The model under review builds one solid part; all positions refer to its coordinate system, in mm. A direction names the side the tool comes from. Round coordinates to 2 decimals unless told otherwise and drop trailing zeros. Write each loop counter-clockwise with the first axis right and the second up, starting at its lowest first coordinate (ties: lowest second). Pieces come first, ordered by that corner, then holes. Notation, with made-up numbers: (-5.75, 68.25) - (48.25, 68.25) arc R11 cw to (48.25, 84.25) - close; hole circle Ø2 at (14.5, -17.5). An arc over 180 degrees is marked (long way). One line per question, with ' | ' between items. Start each with the question number.
```python
from build123d import *

# Parameters (mm, degrees)
F0_R = 31.75
F2_R = 42.4803799305
F4_T = -7.62
F5_R = 5.08
F6_R = 5.08
F7_R = 5.08


with BuildPart() as f3:
    # F0 (on Top) → F3 section 0
    with BuildSketch(Plane.XY):
        Circle(F0_R)
    # F2 (on offset) → F3 section 1
    with BuildSketch(Plane.XY.offset(152.4)):
        Circle(F2_R)
    loft()

    # F4
    f4_openings = [f3.faces().sort_by_distance(p)[0] for p in [
        (0, 0, 152.4),
    ]]
    offset(amount=F4_T, openings=f4_openings, kind=Kind.INTERSECTION)

    # F5
    f5_edges = [f3.edges().sort_by_distance(p)[0] for p in [
        (-42.48038, 0, 152.4),
    ]]
    fillet(f5_edges, radius=F5_R)

    # F6
    f6_edges = [f3.edges().sort_by_distance(p)[0] for p in [
        (-31.75, 0, 0),
    ]]
    fillet(f6_edges, radius=F6_R)

    # F7
    f7_edges = [f3.edges().sort_by_distance(p)[0] for p in [
        (-24.647654, 0, 7.62),
    ]]
    fillet(f7_edges, radius=F7_R)


solid = f3.part
```
1. The part is to be moulded in two halves that separate along X. For faces 1 (the face through (-8.056, -36.277, 76.839)), 2 (the face through (28.6, 9, 83.4)), 3 (the face through (0, 0, 0)), say which applies: pulls with the +X half, pulls with the -X half, needs draft (parallel to the pull), parting line crosses it, or undercut.
2. Clearance check with flat-ended pins moving along their axes: P1, Ø10, axis at y = -18.5, z = 58.5, coming from the +X side; P2, Ø5, axis at y = -17, z = 111.5, coming from the -X side; P3, Ø6, axis at y = -27.5, z = 93, coming from the -X side. State where each tip first meets the part, or that it passes through.
3. Wall thickness on line 1 along Z through (x, y) = (-17, 4); line 2 along X through (y, z) = (4, 78); line 3 along Y through (x, z) = (19.5, 15.5): over which ranges is each line inside the solid? List them lowest first. Write a range as [from, to].
4. Add section A-A, the plane x = 0. Write out the cut boundary in (y, z).
5. Add section B-B, the plane z = 61.5. Write out the cut boundary in (x, y).
6. Add section C-C, the plane z = 41.5. Write out the cut boundary in (x, y), then the cut area to 3 significant figures.
7. Machinability: for faces 4 (the face through (-25, -25, 152.4)), 5 (the face through (0, 0, 7.62)), which of the approach directions +Z, -Z, +X, -X, +Y, -Y give a long, thin tool a straight path to every point of the face, cutting with its end or side? Answer none if there is none.
Geometry check:
1) face 1: parting line crosses it | face 2: undercut | face 3: needs draft
2) P1: stops at x = 33.27 | P2: stops at x = -36.87 | P3: stops at x = -29.45
3) line 1: z = [0, 7.62] | line 2: x = [-37.03, -29.33], [29.33, 37.03] | line 3: y = [-26.43, -15.97], [15.97, 26.43]
4) outline: (-42.1, 146.96) - (-32.08, 4.72) arc R5.08 ccw to (-27.02, 0) - (27.02, 0) arc R5.08 ccw to (32.08, 4.72) - (42.1, 146.96) arc R5.08 ccw to (37.03, 152.4) - (34.84, 152.4) - (24.98, 12.34) arc R5.08 cw to (19.91, 7.62) - (-19.91, 7.62) arc R5.08 cw to (-24.98, 12.34) - (-34.84, 152.4) - (-37.03, 152.4) arc R5.08 ccw to start
5) outline: circle Ø72.16 at (0, 0); hole circle Ø56.88 at (0, 0)
6) outline: circle Ø69.34 at (0, 0); hole circle Ø54.07 at (0, 0) | area: 1,480 mm2
7) face 4: +Z, +X, -X, +Y, -Y | face 5: +Z
